from build123d import *

# Parameters (mm, degrees)
F0_R     = 9
F1_DEPTH = 4
F3_W     = 3
F3_H     = 3
F4_DEPTH = 2
F2_R     = 9
F2_R_2   = 8
F5_DEPTH = 1
F7_DEPTH = 1


# Not quite as in the source:
# - a feature names something its author has since deleted; it is built from what else it names


with BuildPart() as f1:
    # F0 (on Top) → F1 (new body)
    with BuildSketch(Plane.XY):
        with Locations((-31.3306450844, 19.7580661625)):
            Circle(F0_R)
    extrude(amount=F1_DEPTH)

    # F3 (on face) → F4 (cut)
    with BuildSketch(Plane(origin=(0, 0, 0), x_dir=(1, 0, 0), z_dir=(0, 0, -1))):
        with BuildLine():
            ThreePointArc((-32.8306450844, -28.6321858371), (-32.0832814269, -28.7265408676), (-31.3306450844, -28.7580661625))
            ThreePointArc((-31.3306450844, -28.7580661625), (-30.5780087419, -28.7265408676), (-29.8306450844, -28.6321858371))
            Line((-29.8306450844, -28.6321858371), (-29.8306450844, -21.2580661625))
            Line((-29.8306450844, -21.2580661625), (-32.8306450844, -21.2580661625))
            Line((-32.8306450844, -21.2580661625), (-32.8306450844, -28.6321858371))
        make_face()
        with BuildLine():
            ThreePointArc((-40.204764759, -18.2580661625), (-40.2991197895, -19.0054298199), (-40.3306450844, -19.7580661625))
            ThreePointArc((-40.3306450844, -19.7580661625), (-40.2991197895, -20.510702505), (-40.204764759, -21.2580661625))
            Line((-40.204764759, -21.2580661625), (-32.8306450844, -21.2580661625))
            Line((-32.8306450844, -21.2580661625), (-32.8306450844, -18.2580661625))
            Line((-32.8306450844, -18.2580661625), (-40.204764759, -18.2580661625))
        make_face()
        with Locations((-31.3306450844, -19.7580661625)):
            Rectangle(F3_W, F3_H)
        with BuildLine():
            Line((-29.8306450844, -18.2580661625), (-29.8306450844, -21.2580661625))
            Line((-29.8306450844, -21.2580661625), (-22.4565254097, -21.2580661625))
            ThreePointArc((-22.4565254097, -21.2580661625), (-22.3621703793, -20.510702505), (-22.3306450844, -19.7580661625))
            ThreePointArc((-22.3306450844, -19.7580661625), (-22.3621703793, -19.0054298199), (-22.4565254097, -18.2580661625))
            Line((-22.4565254097, -18.2580661625), (-29.8306450844, -18.2580661625))
        make_face()
        with BuildLine():
            Line((-32.8306450844, -10.8839464878), (-32.8306450844, -18.2580661625))
            Line((-32.8306450844, -18.2580661625), (-29.8306450844, -18.2580661625))
            Line((-29.8306450844, -18.2580661625), (-29.8306450844, -10.8839464878))
            ThreePointArc((-29.8306450844, -10.8839464878), (-30.5780087419, -10.7895914574), (-31.3306450844, -10.7580661625))
            ThreePointArc((-31.3306450844, -10.7580661625), (-32.0832814269, -10.7895914574), (-32.8306450844, -10.8839464878))
        make_face()
    extrude(amount=-F4_DEPTH, mode=Mode.SUBTRACT)

    # F2 (on face) → F5 (join)
    with BuildSketch(Plane.XY.offset(4)):
        with Locations((-31.3306450844, 19.7580661625)):
            Circle(F2_R)
        with Locations((-31.3306450844, 19.7580661625)):
            Circle(F2_R_2, mode=Mode.SUBTRACT)
    extrude(amount=F5_DEPTH)

    # F6 (on face) → F7 (join)
    with BuildSketch(Plane.XY.offset(4)):
        Polygon((-34.9050166448, 20.6202120843), (-34.6433972716, 20.9240779367), (-34.5026717981, 20.3743209936), (-34.4223662395, 19.6491017819), (-34.4207141089, 18.7433737938), (-34.5142607427, 17.652222692), (-34.6425682025, 16.9327949487), (-34.7957417285, 16.2514322926), (-34.8255401553, 15.620582776), (-34.5142607427, 15.0062852041), (-34.4480313361, 14.930120185), (-34.2493371085, 14.8407080829), (-34.0506428809, 15.0857628952), (-33.9247925897, 15.6238930448), (-33.8585631831, 16.2381852097), (-33.8179988731, 18.9329782997), (-33.7062427572, 20.331275484), (-33.6789195223, 20.6260155682), (-33.7426497061, 20.8346225789), (-34.1532852441, 21.2949361796), (-34.2956868792, 21.4108256257), (-33.6996102042, 22.3869043351), (-32.9611258864, 23.7554691778), (-32.7839634252, 24.124705329), (-32.7028348052, 24.2952051983), (-32.9478788035, 24.5899452825), (-33.2119733685, 24.7132843353), (-33.4479276451, 24.8085071305), (-33.7319078538, 24.8383055573), (-33.9115455069, 24.8350012963), (-34.0017938873, 24.7356331554), (-33.9877177353, 24.6164394483), (-33.9810851823, 23.9450136062), (-34.1797794099, 23.1461033657), (-34.6028329616, 22.2081137744), (-35.2692903966, 21.1160855415), (-35.3305513962, 21.0697658095), (-35.3355198033, 21.0266902611), (-36.0085977758, 20.1789490503), (-37.0144827221, 19.0496908072), (-37.0782297275, 18.9685621872), (-36.9648088648, 18.947048444), (-36.6833260766, 19.0364677553), (-36.2677239339, 19.31379138), (-35.7353954658, 19.7600288287), (-35.1037108724, 20.357763642), align=None)
        Polygon((-29.9310764641, 19.9206399459), (-30.0105589614, 17.0097722153), (-31.1588076939, 16.8475089676), (-32.3451815909, 16.7018030715), (-32.5140773917, 16.6256428585), (-32.4081067365, 16.4567530655), (-31.9974772062, 16.2150073205), (-31.5239165226, 16.2017602376), (-29.45586365, 16.4940071067), (-26.5731061692, 16.6256428585), (-26.3976198696, 16.6256428585), (-26.2519319967, 16.7282972372), (-26.2618447798, 16.8756552638), (-26.3943156085, 17.059450278), (-27.1311057416, 17.4096598934), (-27.8447660474, 17.3806665048), (-28.563352706, 17.2415931617), (-29.3581176009, 17.1124326018), (-29.3291602587, 18.5935345676), (-29.2555052764, 20.0365474153), (-28.8018001977, 20.1027828296), (-28.1179983962, 20.1897209413), (-27.2114293234, 20.297343727), (-26.0862984027, 20.4239990563), (-25.9414516145, 20.4223409181), (-25.791618396, 20.5895845884), (-25.8826958455, 20.7419230375), (-26.1127925684, 20.9372949808), (-26.746970377, 21.103709582), (-27.5368089191, 21.0001960954), (-28.2669905301, 20.8387679245), (-28.7885831536, 20.731139131), (-29.1114394953, 20.6657327858), (-29.2422281548, 20.629325837), (-29.1661099961, 22.4531697882), (-28.8978640776, 24.103137516), (-28.9649105379, 24.2819881542), (-29.1661099961, 24.5137670463), (-29.6983964099, 24.7356331554), (-30.1131712858, 24.858191201), (-30.3367195641, 24.8408288112), (-30.4973066504, 24.7687959206), (-30.5701806256, 24.6048444959), (-30.4840896063, 24.4110946444), (-30.1521014886, 23.8050931708), (-30.0237760055, 23.3182854043), (-29.9790783653, 21.9216643815), (-29.9310764641, 20.500165277), (-31.318589742, 20.331275484), (-32.9346317206, 20.1921961332), (-33.203712716, 20.0646937115), (-33.0372981148, 19.8709618832), (-32.5910546583, 19.5845245058), (-32.2027799559, 19.5232514908), (-32.0107242891, 19.5629927394), (-31.5628287021, 19.6507539124), (-30.8673838862, 19.7741049807), align=None)
    extrude(amount=F7_DEPTH)


solid = f1.part
Source: CAD feature listing. Evaluate the final solid. Frame: model axes, mm. A direction names the side the tool comes from. Round coordinates to 2 decimals unless told otherwise and drop trailing zeros. Loops run counter-clockwise (first coordinate to the right, second up) from the corner with the lowest first, then second, coordinate; pieces in that order, holes last. Notation, with made-up numbers: (35, 62.5) - (85, 62.5) arc R30 cw to (85, 96.5) - close; hole circle Ø1 at (-12, -27). An arc over 180 degrees is marked (long way). Write item = value, one per line. Start each with the question number.
Item 1: Section query A-A on y = 25.75. Output: boundary loops of the cut face in (x, z), plus the area to 3 significant figures.
Item 2: Mould query, pull axis X, two halves, no side actions, for faces 1 (the face through (-29.831, 15, 1)), 2 (the face through (-36, 24, 0)), 3 (the face through (-32, 20, 2)). Classes: released by +X, released by -X, zero draft, split by the parting line, or undercut.
Item 3: First-contact query: pin 1 Ø1 at (x, z) = (-27.5, 2.5) entering from -Y; pin 2 Ø2 at (y, z) = (24, 1.5) entering from +X; pin 3 Ø0.6 at (x, z) = (-37, 1) entering from +Y. Flat tips, straight axial feed; report the tip coordinate or a pass-through.
Item 4: Section query C-C on x = -37.5. Output: boundary loops of the cut face in (y, z).
Item 5: Section query B-B on z = 4.6. Count the separate pieces of the cut face and the enclosed holes in it, plus the area to 3 significant figures.
Item 6: Material intervals for line 1 (Y direction, x = -28.5, z = 4.3); line 2 (Z direction, x = -28.75, y = 17.5); line 3 (Y direction, x = -24.5, z = 0.6), sorted ascending.
Item 7: Section query D-D on z = 3.15. Output: boundary loops of the cut face in (x, y).
Item 8: Reachability of faces 4 (the face through (-39, 16, 5)), 5 (the face through (-29.831, 25, 1)), 6 (the face through (-33.336, 23.062, 4.493)) from +Z, -Z, +X, -X, +Y, -Y: full face, straight path, thin tool, end or side. Return the list, or none.
Results list:
q1.outline = (-38.05, 0) - (-32.83, 0) - (-32.83, 2) - (-29.83, 2) - (-29.83, 0) - (-24.62, 0) - (-24.62, 5) - (-26.03, 5) - (-26.03, 4) - (-36.63, 4) - (-36.63, 5) - (-38.05, 5) - close
q1.area = 50.6 mm²
q2.face_1 = undercut
q2.face_2 = zero draft
q2.face_3 = undercut
q3.pin_1 = 11.4
q3.pin_2 = -22.93
q3.pin_3 = 26.98
q4.outline = (13.21, 0) - (18.26, 0) - (18.26, 2) - (21.26, 2) - (21.26, 0) - (26.31, 0) - (26.31, 5) - (24.85, 5) - (24.85, 4) - (14.67, 4) - (14.67, 5) - (13.21, 5) - close
q5.separate_pieces = 3
q5.enclosed_holes = 1
q5.area = 77.2 mm²
q6.line_1 = 11.21 to 12.28, 16.54 to 17.25, 20.14 to 20.79, 27.24 to 28.3
q6.line_2 = 0 to 4
q6.line_3 = 13.9 to 18.26, 21.26 to 25.62
q7.outline = circle Ø18 at (-31.33, 19.76)
q8.face_4 = +Z, +X, -X, +Y, -Y
q8.face_5 = -Z, +Y, -Y
q8.face_6 = +Z
